```python
from build123d import *

# Parameters (mm, degrees)
BOSS_EXTRUDE1_DEPTH = 25.4
CUT_EXTRUDE1_START  = -15.875
CUT_EXTRUDE1_DEPTH  = 15.875


with BuildPart() as part:
    # Sketch1 → Boss-Extrude1 (new body)
    with BuildSketch(Plane.YZ):
        with BuildLine():
            Line((0, 0), (44.42968, 0))
            Line((44.42968, 0), (44.42968, -19.05))
            Line((44.42968, -19.05), (19.05, -19.05))
            Line((19.05, -19.05), (19.05, -59.6646))
            Line((19.05, -59.6646), (84.99856, -59.6646))
            Line((84.99856, -59.6646), (84.99856, -19.05))
            Line((84.99856, -19.05), (59.61888, -19.05))
            Line((59.61888, -19.05), (59.61888, 0))
            Line((59.61888, 0), (104.04856, 0))
            Line((104.04856, 0), (104.04856, -81.8896))
            Line((104.04856, -81.8896), (58.34888, -81.8896))
            Line((58.34888, -81.8896), (58.34888, -100.9396))
            ThreePointArc((58.34888, -100.9396), (52.02428, -124.652748271), (45.69968, -100.9396))
            Line((45.69968, -100.9396), (45.69968, -81.8896))
            Line((45.69968, -81.8896), (0, -81.8896))
            Line((0, -81.8896), (0, 0))
        make_face()
    extrude(amount=BOSS_EXTRUDE1_DEPTH)

    # Sketch2 → Cut-Extrude1 (cut)
    with BuildSketch(Plane.YZ.offset(25.4).offset(CUT_EXTRUDE1_START)):
        with BuildLine():
            Line((45.69968, -81.8896), (58.34888, -81.8896))
            Line((58.34888, -81.8896), (58.34888, -100.9396))
            ThreePointArc((58.34888, -100.9396), (52.02428, -99.252748271), (45.69968, -100.9396))
            Line((45.69968, -100.9396), (45.69968, -81.8896))
        make_face()
    extrude(amount=CUT_EXTRUDE1_DEPTH, mode=Mode.SUBTRACT)


solid = part.part
```
Could you check a few things on this model? Use its own coordinates, in mm. A direction names the side the tool comes from. Coordinates: 2 decimals unless noted, no trailing zeros. Write each loop counter-clockwise with the first axis right and the second up, starting at its lowest first coordinate (ties: lowest second). Pieces come first, ordered by that corner, then holes. Notation, with made-up numbers: (6, 82) -> (58, 82) arc R19 ccw to (58, 102) -> close; hole circle Ø5 at (62.5, 63.5). An arc over 180 degrees is marked (long way). One line per question, with ' | ' between items. Start each with the question number.
1. Will these pins go through, and if not, where does the flat tip stop? P1, Ø2, axis at x = 19.5, z = -58, coming from the -Y side; P2, Ø1.5, axis at x = 15.5, z = -108.5, coming from the -Y side; P3, Ø10, axis at x = 13, y = 70.5, coming from the -Z side; P4, Ø5, axis at x = 3, z = -93.5, coming from the -Y side.
2. Thinking about a two-plate mould opening in Y: for faces 1 (the face through (13, 0, -42)), 2 (the face through (13, 72, -19.05)), 3 (the face through (9.525, 52, -91)), 4 (the face through (13, 44.43, -9)), which applies, pulls with the +Y half, pulls with the -Y half, needs draft (parallel to the pull), parting line crosses it, or undercut?
3. Please list where these lines run through material, in increasing order: line 1 along Y through (x, z) = (16.25, -53); line 2 along Z through (x, y) = (4.5, 30); line 3 along Z through (x, y) = (4.5, 63.5).
4. For faces 5 (the face through (13, 59.619, -10)), 6 (the face through (5, 45.7, -92)), 7 (the face through (13, 19.05, -39)), 8 (the face through (5, 58.349, -91)), which set-ups out of +Z, -Z, +X, -X, +Y, -Y let a thin tool reach every point of the face, with its end or its side?
5. If we section it at D-D (x = 5): Please give me the cut outline in (y, z), and give its area (3 significant figures).
6. If we section it at A-A (x = 17.5): Please give me the cut outline in (y, z), and give its area (3 significant figures).
7. If we section it at B-B (z = -10): Please give me the cut outline in (x, y), and give its area (3 significant figures).
8. If we section it at C-C (y = 26): Please give me the cut outline in (x, z), and give its area (3 significant figures).
Return value:
1) P1: stops at y = 0 | P2: stops at y = 39.62 | P3: stops at z = -81.89 | P4: stops at y = 45.7
2) face 1: pulls with the -Y half | face 2: undercut | face 3: needs draft | face 4: undercut
3) line 1: y = 0 to 19.05, 85 to 104.05 | line 2: z = -81.89 to -59.66, -19.05 to 0 | line 3: z = -117.39 to -106.51, -81.89 to -59.66, -19.05 to 0
4) face 5: +Z, +X, -X | face 6: +X, -X, -Y | face 7: +X, -X | face 8: +X, -X, +Y
5) outline: (0, -81.89) -> (45.7, -81.89) -> (45.7, -100.94) arc R12.7 ccw (long way) to (58.35, -100.94) -> (58.35, -81.89) -> (104.05, -81.89) -> (104.05, 0) -> (59.62, 0) -> (59.62, -19.05) -> (85, -19.05) -> (85, -59.66) -> (19.05, -59.66) -> (19.05, -19.05) -> (44.43, -19.05) -> (44.43, 0) -> (0, 0) -> close | area: 6,290 mm²
6) outline: (0, -81.89) -> (104.05, -81.89) -> (104.05, 0) -> (59.62, 0) -> (59.62, -19.05) -> (85, -19.05) -> (85, -59.66) -> (19.05, -59.66) -> (19.05, -19.05) -> (44.43, -19.05) -> (44.43, 0) -> (0, 0) -> close; circle Ø25.4 at (52.02, -111.95) | area: 6,060 mm²
7) outline: (0, 0) -> (25.4, 0) -> (25.4, 44.43) -> (0, 44.43) -> close; (0, 59.62) -> (25.4, 59.62) -> (25.4, 104.05) -> (0, 104.05) -> close | area: 2,260 mm²
8) outline: (0, -81.89) -> (25.4, -81.89) -> (25.4, -59.66) -> (0, -59.66) -> close; (0, -19.05) -> (25.4, -19.05) -> (25.4, 0) -> (0, 0) -> close | area: 1,050 mm²
